Could you check a few things on this model? Use its own coordinates, in mm. Face numbers are marked on the shaded views. A direction names the side the tool comes from. Round coordinates to 2 decimals unless told otherwise and drop trailing zeros. Write each loop counter-clockwise with the first axis right and the second up, starting at its lowest first coordinate (ties: lowest second). Pieces come first, ordered by that corner, then holes. Notation, with made-up numbers: (5, 52) -> (52, 52) arc R18 cw to (52, 56) -> close; hole circle Ø1 at (-22.75, 18.5). An arc over 180 degrees is marked (long way). Answer in a Markdown table with one row per item. Add a question column.
```python
from build123d import *

# Parameters (mm, degrees)
F1_DEPTH = 12.7
F2_R     = 3.175
F3_DEPTH = 25.4
F4_W     = 12.7
F4_H     = 25.4
F5_DEPTH = 12.7
F6_W     = 12.7
F6_H     = 12.7
F7_DEPTH = 6.35


with BuildPart() as f1:
    # F0 (on Front) → F1 (new body)
    with BuildSketch(Plane.XZ):
        with BuildLine():
            Line((-12.7, -12.7), (0, -12.7))
            ThreePointArc((0, -12.7), (12.7, 0), (0, 12.7))
            Line((0, 12.7), (-12.7, 12.7))
            Line((-12.7, 12.7), (-12.7, -12.7))
        make_face()
    extrude(amount=F1_DEPTH)

    # F2 (on face) → F3 (cut)
    with BuildSketch(Plane.XZ.offset(12.7)):
        Circle(F2_R)
    extrude(amount=-F3_DEPTH, mode=Mode.SUBTRACT)

    # F4 (on face) → F5 (join)
    with BuildSketch(Plane(origin=(-12.7, 0, 0), x_dir=(0, -1, 0), z_dir=(-1, 0, 0))):
        with Locations((6.35, 0)):
            Rectangle(F4_W, F4_H)
        with Locations((19.05, 0)):
            Rectangle(F4_W, F4_H)
    extrude(amount=F5_DEPTH)

    # F6 (on face) → F7 (cut)
    with BuildSketch(Plane.XZ.offset(25.4)):
        with Locations((-19.05, 0)):
            Rectangle(F6_W, F6_H)
    extrude(amount=-F7_DEPTH, mode=Mode.SUBTRACT)


solid = f1.part
```
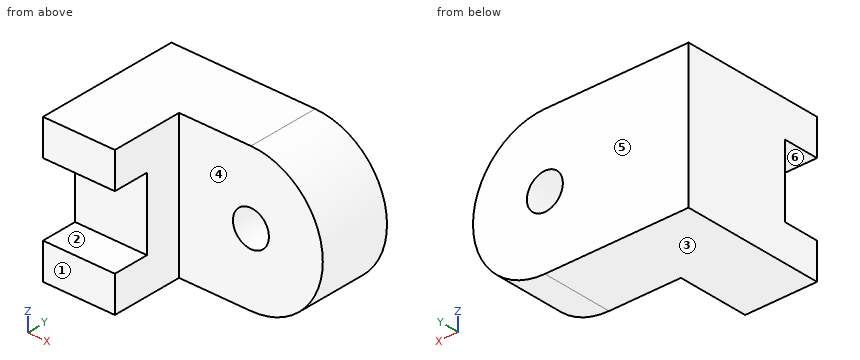
(1) If we mould it in two halves opening along Z, with no side actions, what happens to the marked faces 1, 2 and 3? For each: pulls with the +Z half, pulls with the -Z half, needs draft (parallel to the pull), parting line crosses it, or undercut.
(2) I need wall thicknesses on L1, parallel to Z at x = -19, y = -21.5; L2, parallel to Y at x = 9.5, z = 1; L3, parallel to Y at x = -22, z = -5.5. Which ranges of each line are inside material? Lowest first, please.
(3) Suppose I cut it at C-C, the plane x = -16.5. Please give me the cut outline in (y, z), then the cut area to 3 significant figures.
(4) For P1, Ø6, axis at x = -3, z = 2, coming from the -Y side; P2, Ø3, axis at y = -9, z = -2.5, coming from the +X side; P3, Ø6.5, axis at y = -19.5, z = -2, coming from the +X side, each with a flat end and sliding along its axis, tell me the tip position at first contact or that it passes through.
(5) Suppose I cut it at A-A, the plane y = -22.5. Please give me the cut outline in (x, z).
(6) Suppose I cut it at D-D, the plane y = -16.25. Please give me the cut outline in (x, z), then the cut area to 3 significant figures.
(7) Suppose I cut it at B-B, the plane z = 0. Please give me the cut outline in (x, y) (3 decimals), then the cut area to 3 significant figures.
(8) On a 3-axis mill with a long thin cutter (end or side, diameter ignored), from which of +Z, -Z, +X, -X, +Y, -Y can I reach the whole of each face in a straight line? I mean the marked faces 4, 5 and 6. Say none if no direction works.
Response:
| question | item | result |
|---|---|---|
| 1 | face 1 | needs draft |
| 1 | face 2 | undercut |
| 1 | face 3 | pulls with the -Z half |
| 2 | L1 | -12.7 to -6.35, 6.35 to 12.7 |
| 2 | L2 | -12.7 to 0 |
| 2 | L3 | -19.05 to 0 |
| 3 | outline | (-25.4, -12.7) -> (0, -12.7) -> (0, 12.7) -> (-25.4, 12.7) -> (-25.4, 6.35) -> (-19.05, 6.35) -> (-19.05, -6.35) -> (-25.4, -6.35) -> close |
| 3 | area | 565 mm² |
| 4 | P1 | y = -12.7 |
| 4 | P2 | x = 12.66 |
| 4 | P3 | x = -12.7 |
| 5 | outline | (-25.4, -12.7) -> (-12.7, -12.7) -> (-12.7, -6.35) -> (-25.4, -6.35) -> close; (-25.4, 6.35) -> (-12.7, 6.35) -> (-12.7, 12.7) -> (-25.4, 12.7) -> close |
| 6 | outline | (-25.4, -12.7) -> (-12.7, -12.7) -> (-12.7, 12.7) -> (-25.4, 12.7) -> close |
| 6 | area | 323 mm² |
| 7 | outline | (-25.4, -19.05) -> (-12.7, -19.05) -> (-12.7, -12.7) -> (-3.175, -12.7) -> (-3.175, 0) -> (-25.4, 0) -> close; (3.175, -12.7) -> (12.7, -12.7) -> (12.7, 0) -> (3.175, 0) -> close |
| 7 | area | 484 mm² |
| 8 | face 4 | +Z, -Z, +X, -Y |
| 8 | face 5 | +Z, -Z, +X, -X, +Y |
| 8 | face 6 | +X, -X, -Y |
